Geometry check sheet. Reference: the model listing, model coordinates, mm. A direction names the side the tool comes from. Round coordinates to 2 decimals unless told otherwise and drop trailing zeros. Order: outer loops, then holes, each group sorted by start corner. A loop starts at its lowest first (then second) coordinate and runs counter-clockwise, first axis right, second up.
```python
from build123d import *

# Parameters (mm, degrees)
F0_W     = 7.9375
F0_H     = 358.775
F0_R     = 2.15265
F1_DEPTH = 6.35
F2_W     = 7.9375
F2_H     = 3.175
F3_DEPTH = 7.9375
F4_R     = 0.762


with BuildPart() as f1:
    # F0 (on Top) → F1 (new body)
    with BuildSketch(Plane.XY):
        Rectangle(F0_W, F0_H)
        with Locations((0, -173.83125)):
            Circle(F0_R, mode=Mode.SUBTRACT)
        with Locations((0, 173.83125)):
            Circle(F0_R, mode=Mode.SUBTRACT)
    extrude(amount=F1_DEPTH)

    # F2 (on face) → F3 (cut, through all)
    with BuildSketch(Plane.YZ.offset(3.96875)):
        with Locations((0, 1.5875)):
            Rectangle(F2_W, F2_H)
    extrude(amount=-F3_DEPTH, mode=Mode.SUBTRACT)

    # F4
    f4_edges = [f1.edges().sort_by_distance(p)[0] for p in [
        (0, -179.3875, 0),
        (3.96875, -91.678125, 0),
        (3.96875, 91.678125, 0),
        (-3.96875, 91.678125, 0),
        (-3.96875, -91.678125, 0),
        (0, 179.3875, 0),
        (-3.96875, 0, 6.35),
        (0, -179.3875, 6.35),
        (3.96875, 0, 6.35),
        (0, 179.3875, 6.35),
    ]]
    fillet(f4_edges, radius=F4_R)


solid = f1.part
```
(1) Material ranges on line 1 (Y direction, x = 0, z = 3.25); line 2 (Y direction, x = 0, z = 3); line 3 (Y direction, x = 3.25, z = 2), recorded low to high.
Returned:
line 1: y = -179.39 to -175.98, -171.68 to 171.68, 175.98 to 179.39
line 2: y = -179.39 to -175.98, -171.68 to -3.97, 3.97 to 171.68, 175.98 to 179.39
line 3: y = -179.39 to -3.97, 3.97 to 179.39
(2) Sectioned sample at B-B, the plane z = 1.75. Record the cut outline in (x, y).
Returned:
outline: (-3.97, -179.39) - (3.97, -179.39) - (3.97, -3.97) - (-3.97, -3.97) - close; (-3.97, 3.97) - (3.97, 3.97) - (3.97, 179.39) - (-3.97, 179.39) - close; hole circle Ø4.31 at (0, -173.83); hole circle Ø4.31 at (0, 173.83)
(3) Sectioned sample at A-A, the plane x = 0. Give the number of separate pieces and of enclosed holes in the cut face, and give its area (3 significant figures).
Returned:
separate pieces: 3
enclosed holes: 0
area: 2,200 mm2
(4) Set-up check for faces 1 (the flat face through (0, -90, 0)), 2 (the flat face through (0, 0, 3.175)): record each of +Z, -Z, +X, -X, +Y, -Y from which the full face is reachable in a straight line by a thin tool's end or side.
Returned:
face 1: -Z, +X, -X, +Y, -Y
face 2: -Z, +X, -X
